For this review, use the dimensioned drawing (mm, ordinates from the lowest corner) and the shaded views. A direction names the side the tool comes from. Round coordinates to 2 decimals unless told otherwise and drop trailing zeros. Write each loop counter-clockwise with the first axis right and the second up, starting at its lowest first coordinate (ties: lowest second). Pieces come first, ordered by that corner, then holes.
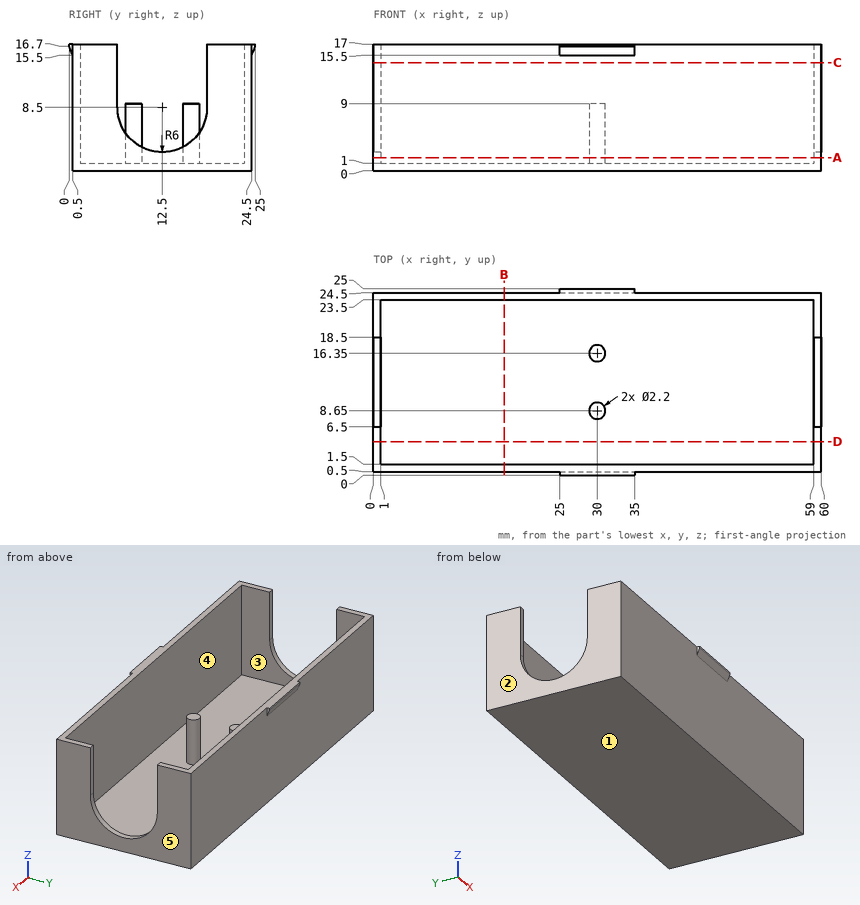
(1) We need section C-C, the plane z = 14.5. Give the boundary of the cut face in (x, y), and give its area (3 significant figures).
Geometry check:
outline: (0, 0.5) - (60, 0.5) - (60, 6.5) - (59, 6.5) - (59, 1.5) - (1, 1.5) - (1, 6.5) - (0, 6.5) - close; (0, 18.5) - (1, 18.5) - (1, 23.5) - (59, 23.5) - (59, 18.5) - (60, 18.5) - (60, 24.5) - (0, 24.5) - close
area: 140 mm2
(2) Mouldability with a two-part tool opening along X and no side actions: class the marked faces 1, 2 and 3 as pulls with the +X half, pulls with the -X half, needs draft (parallel to the pull), parting line crosses it, or undercut.
Geometry check:
face 1: needs draft
face 2: pulls with the -X half
face 3: undercut
(3) For line 1 along X through (y, z) = (19.5, 2.5); line 2 along Y through (x, z) = (15.5, 13.25); line 3 along Z through (x, y) = (10, 1.75), list the stretches that pass through material, from the lowest coordinate up.
Geometry check:
line 1: x = 0 to 1, 59 to 60
line 2: y = 0.5 to 1.5, 23.5 to 24.5
line 3: z = 0 to 1
(4) We need section A-A, the plane z = 1.75. Give the boundary of the cut face in (x, y).
Geometry check:
outline: (0, 0.5) - (60, 0.5) - (60, 24.5) - (0, 24.5) - close; circle Ø2.2 at (30, 8.65); circle Ø2.2 at (30, 16.35); hole (1, 1.5) - (59, 1.5) - (59, 23.5) - (1, 23.5) - close
(5) For pin 1 Ø4 at (x, y) = (11.5, 14) entering from -Z; pin 2 Ø1.8 at (x, y) = (30.5, 16.5) entering from +Z; pin 3 Ø0.6 at (y, z) = (0, 16) entering from +X; pin 4 Ø8 at (x, z) = (21, 7) entering from -Y, all flat-tipped, find the tip position at first contact; note any pin that passes through.
Geometry check:
pin 1: stops at z = 0
pin 2: stops at z = 9
pin 3: stops at x = 35
pin 4: stops at y = 0.5
(6) For the marked faces 4 and 5, list the 3-axis set-ups (+Z, -Z, +X, -X, +Y, -Y) from which the entire face can be reached by the end or side of a thin tool; tool diameter is ignored.
Geometry check:
face 4: +Z
face 5: +Z, -Z, +X, +Y, -Y
(7) We need section B-B, the plane x = 17.5. Give the boundary of the cut face in (y, z), and give its area (3 significant figures).
Geometry check:
outline: (0.5, 0) - (24.5, 0) - (24.5, 17) - (23.5, 17) - (23.5, 1) - (1.5, 1) - (1.5, 17) - (0.5, 17) - close
area: 56.0 mm2
(8) We need section D-D, the plane y = 4.5. Give the boundary of the cut face in (x, z), and give its area (3 significant figures).
Geometry check:
outline: (0, 0) - (60, 0) - (60, 17) - (59, 17) - (59, 1) - (1, 1) - (1, 17) - (0, 17) - close
area: 92.0 mm2
